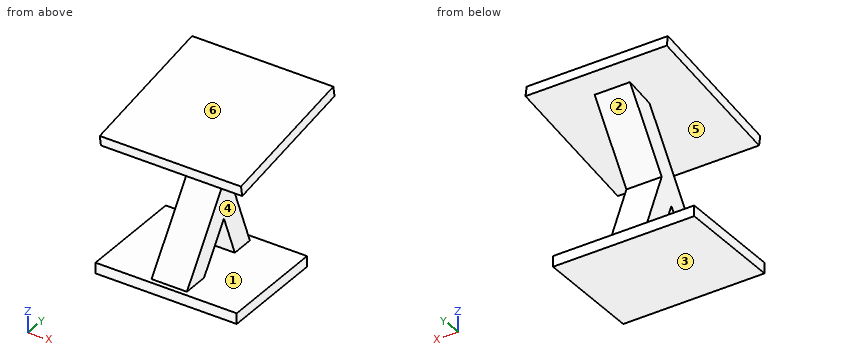
from build123d import *

# Parameters (mm, degrees)
BOSS_EXTRUDE1_DEPTH = 5
SKETCH3_W           = 3
SKETCH3_H           = 30
BOSS_EXTRUDE2_DEPTH = 20


with BuildPart() as part:
    # Sketch2 → Boss-Extrude1 (new, symmetric)
    with BuildSketch(Plane(origin=(0, 0, 0), x_dir=(0, 0, -1), z_dir=(1, 0, 0))):
        Polygon((-3, -98.903535581), (-3, -92.474380652), (-21.018302161, -99.410083352), (-40.334338568, -85.884849051), (-38.860884921, -94.241219935), (-3, -119.351281883), (-3, -112.02663435), (-15.093539832, -103.558646596), align=None)
    extrude(amount=BOSS_EXTRUDE1_DEPTH, both=True)

    # Sketch3 → Boss-Extrude2 (add, symmetric)
    with BuildSketch(Plane(origin=(0, 0, 0), x_dir=(0, 0, -1), z_dir=(1, 0, 0))):
        with Locations((-1.5, -105.688958117)):
            Rectangle(SKETCH3_W, SKETCH3_H)
        Polygon((-44.510684425, -79.475926173), (-37.564757318, -118.868236293), (-34.610334059, -118.34729176), (-41.556261166, -78.95498164), align=None)
    extrude(amount=BOSS_EXTRUDE2_DEPTH, both=True)


solid = part.part
Model file for the job. Use its own axes, mm. Face numbers are marked on the shaded views. A direction names the side the tool comes from. Coordinates: 2 decimals unless noted, no trailing zeros. Order: outer loops, then holes, each group sorted by start corner. A loop starts at its lowest first (then second) coordinate and runs counter-clockwise, first axis right, second up. Notation, with made-up numbers: (28.25, -23.5) -> (70.25, -23.5) arc R24 cw to (70.25, 1.5) -> close; hole circle Ø1 at (65.25, 67). An arc over 180 degrees is marked (long way). Return JSON: item names as keys, results as strings. Group by question number.
Item 1: Saw through at C-C on z = 11. Write the cut outline in (x, y).
Item 2: Pull direction Z, two halves, no side cores. Call the marked faces 3, 4, 5 and 6: pulls with the +Z half, pulls with the -Z half, needs draft (parallel to the pull), parting line crosses it, or undercut.
Item 3: Saw through at D-D on x = -4. Write the cut outline in (y, z).
Item 4: Flat gauge pins, fed straight in: P1, Ø0.9, axis at x = -10, z = 1.5, coming from the +Y side; P2, Ø10, axis at y = -100.5, z = 13.5, coming from the -X side; P3, Ø3, axis at y = -114.5, z = 5.5, coming from the +X side. Where does each tip first touch, or does it go through?
Item 5: Tool access for the marked faces 1 and 2: list every direction of +Z, -Z, +X, -X, +Y, -Y with a clear straight run to the whole face (end or side of a thin tool).
Item 6: Saw through at A-A on x = 8. Write the cut outline in (y, z).
Item 7: Wall check: line 1 along Z through (x, y) = (9, -106.5); line 2 along X through (y, z) = (-97.5, 14); line 3 along Z through (x, y) = (-13.5, -106). Give the ranges that are in metal, low to high. Write a range as [from, to].
Item 8: Saw through at B-B on y = -109. Write the cut outline in (x, z), then the cut area to 3 significant figures.
Values found:
{
 "1": {"outline": "(-5, -113.75) -> (5, -113.75) -> (5, -106.42) -> (-5, -106.42) -> close; (-5, -101.98) -> (5, -101.98) -> (5, -95.55) -> (-5, -95.55) -> close"},
 "2": {"face 3": "pulls with the -Z half", "face 4": "undercut", "face 5": "undercut", "face 6": "pulls with the +Z half"},
 "3": {"outline": "(-120.69, 0) -> (-90.69, 0) -> (-90.69, 3) -> (-92.47, 3) -> (-99.41, 21.02) -> (-85.88, 40.33) -> (-78.95, 41.56) -> (-79.48, 44.51) -> (-118.87, 37.56) -> (-118.35, 34.61) -> (-94.24, 38.86) -> (-119.35, 3) -> (-120.69, 3) -> close; hole (-112.03, 3) -> (-98.9, 3) -> (-103.56, 15.09) -> close"},
 "4": {"P1": "stops at y = -90.69", "P2": "stops at x = -5", "P3": "stops at x = 5"},
 "5": {"face 1": "none", "face 2": "+X, -X, +Y"},
 "6": {"outline": "(-120.69, 0) -> (-90.69, 0) -> (-90.69, 3) -> (-120.69, 3) -> close; (-118.87, 37.56) -> (-118.35, 34.61) -> (-78.95, 41.56) -> (-79.48, 44.51) -> close"},
 "7": {"line 1": "z = [0, 3], [36.7, 39.75]", "line 2": "x = [-5, 5]", "line 3": "z = [0, 3], [36.79, 39.83]"},
 "8": {"outline": "(-20, 0) -> (20, 0) -> (20, 3) -> (-20, 3) -> close; (-20, 36.26) -> (20, 36.26) -> (20, 39.3) -> (-20, 39.3) -> close; (-5, 7.32) -> (5, 7.32) -> (5, 17.78) -> (-5, 17.78) -> close", "area": "346 mm2"}
}
